Drawing for the job (mm, zero at the part's lowest x, y, z). Round coordinates to 2 decimals unless told otherwise and drop trailing zeros. Order: outer loops, then holes, each group sorted by start corner. A loop starts at its lowest first (then second) coordinate and runs counter-clockwise, first axis right, second up. Notation, with made-up numbers: (36.5, 60.25) -> (88.5, 60.25) arc R17 ccw to (88.5, 75.25) -> close; hole circle Ø4 at (-36, 22). An arc over 180 degrees is marked (long way). Answer as CSV lines item,"result". Start each with the question number.
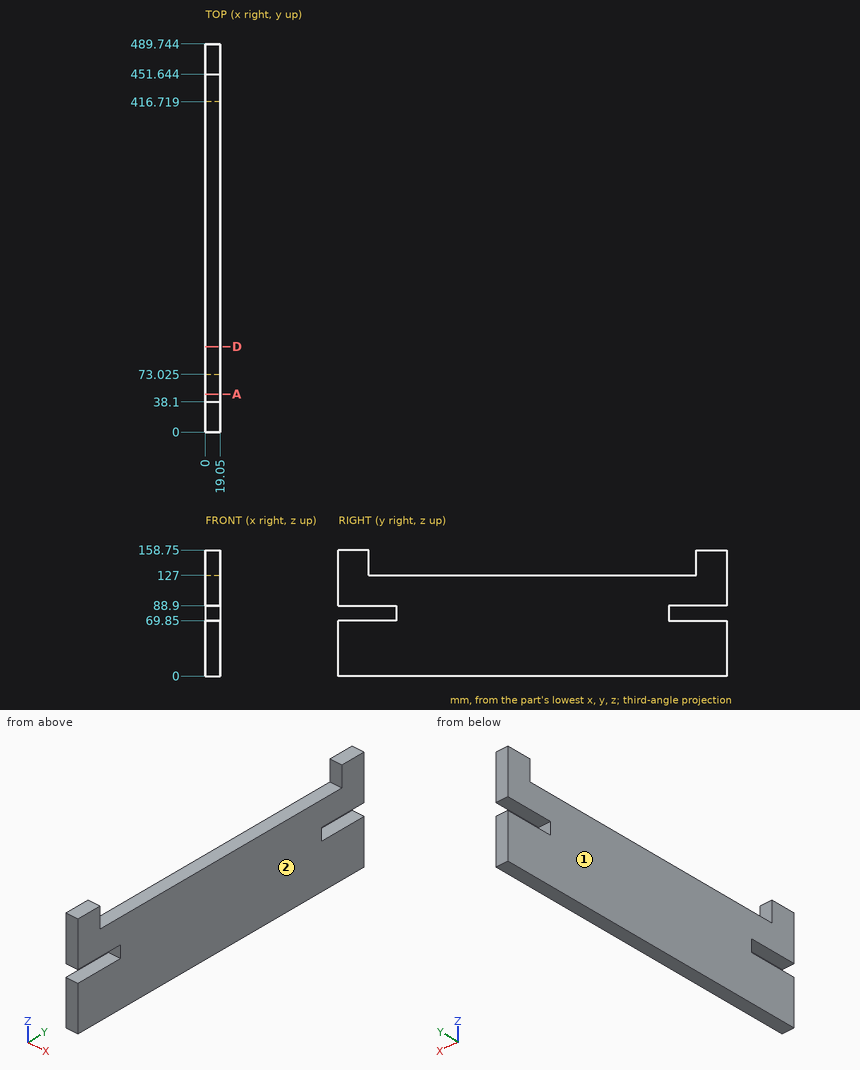
Q1. Slice it at A-A, the plane y = 48. Write the cut outline in (x, z).
Q2. Probe L1, parallel to Y at x = 3.25, z = 140.5; L2, parallel to Z at x = 5.75, y = 440.5; L3, parallel to Z at x = 3, y = 396. List the from-to ranges inside material, lowest first.
Q3. Two-plate mould, pull along X, no slides. Class the marked faces 1 and 2: +X half, -X half, draft (parallel to the pull), parting line (faces both ways), or undercut.
Q4. Slice it at D-D, the plane y = 108. Write the cut outline in (x, z), plus the area to 3 significant figures.
Q5. Flat gauge pins, fed straight in: pin 1 Ø2 at (x, z) = (6, 86) entering from -Y (3 decimals); pin 2 Ø1 at (x, y) = (16.5, 317.5) entering from +Z; pin 3 Ø1 at (x, y) = (2.5, 289.5) entering from -Z; pin 4 Ø5.5 at (x, z) = (9.5, 83.5) entering from +Y. Where does each tip first touch, or does it go through?
Solutions:
1,outline,"(0, 0) -> (19.05, 0) -> (19.05, 69.85) -> (0, 69.85) -> close; (0, 88.9) -> (19.05, 88.9) -> (19.05, 127) -> (0, 127) -> close"
2,L1,"y = 0 to 38.1, 451.64 to 489.74"
2,L2,"z = 0 to 69.85, 88.9 to 127"
2,L3,"z = 0 to 127"
3,face 1,"-X half"
3,face 2,"+X half"
4,outline,"(0, 0) -> (19.05, 0) -> (19.05, 127) -> (0, 127) -> close"
4,area,"2,420 mm2"
5,pin 1,"stops at y = 73.025"
5,pin 2,"stops at z = 127"
5,pin 3,"stops at z = 0"
5,pin 4,"stops at y = 416.72"
